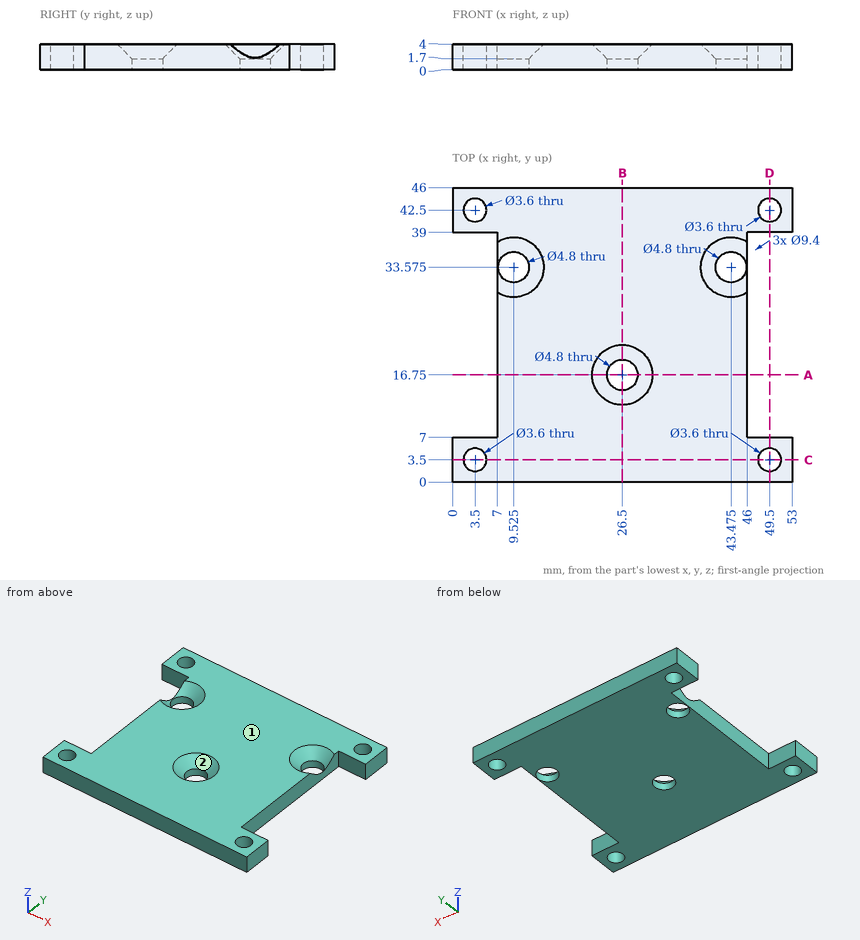
For this review, use the dimensioned drawing (mm, ordinates from the lowest corner) and the shaded views. Coordinates: 2 decimals unless noted, no trailing zeros. Loops run counter-clockwise (first coordinate to the right, second up) from the corner with the lowest first, then second, coordinate; pieces in that order, holes last.
1. For line 1 (Y direction, x = 3.5, z = 0.8); line 2 (X direction, y = 42.5, z = 1.25); line 3 (X direction, y = 4.5, z = 1.8), list the stretches that pass through material, from the lowest coordinate up.
2. Add section D-D, the plane x = 49.5. Give the boundary of the cut face in (y, z).
3. Insertion check: P1, Ø1.2, axis at y = 20.5, z = 2, coming from the +X side; P2, Ø2, axis at y = 27, z = 1.5, coming from the -X side. Each pin has a flat end and moves straight along its axis. Give the tip position at first contact, or say it passes through.
4. Mouldability with a two-part tool opening along Y and no side actions: class the marked faces 1 and 2 as +Y half, -Y half, draft (parallel to the pull), parting line (faces both ways), or undercut.
5. Add section C-C, the plane y = 3.5. Give the boundary of the cut face in (x, z), then the cut area to 3 significant figures.
6. Add section B-B, the plane x = 26.5. Give the boundary of the cut face in (y, z).
7. Add section A-A, the plane y = 16.75. Give the boundary of the cut face in (x, z).
Result:
1. line 1: y = 0 to 1.7, 5.3 to 7, 39 to 40.7, 44.3 to 46
1. line 2: x = 0 to 1.7, 5.3 to 47.7, 51.3 to 53
1. line 3: x = 0 to 2, 5 to 48, 51 to 53
2. outline: (0, 0) - (1.7, 0) - (1.7, 4) - (0, 4) - close; (5.3, 0) - (7, 0) - (7, 4) - (5.3, 4) - close; (39, 0) - (40.7, 0) - (40.7, 4) - (39, 4) - close; (44.3, 0) - (46, 0) - (46, 4) - (44.3, 4) - close
3. P1: stops at x = 46
3. P2: stops at x = 7
4. face 1: draft
4. face 2: undercut
5. outline: (0, 0) - (1.7, 0) - (1.7, 4) - (0, 4) - close; (5.3, 0) - (47.7, 0) - (47.7, 4) - (5.3, 4) - close; (51.3, 0) - (53, 0) - (53, 4) - (51.3, 4) - close
5. area: 183 mm2
6. outline: (0, 0) - (14.35, 0) - (14.35, 1.7) - (12.05, 4) - (0, 4) - close; (19.15, 0) - (46, 0) - (46, 4) - (21.45, 4) - (19.15, 1.7) - close
7. outline: (7, 0) - (24.1, 0) - (24.1, 1.7) - (21.8, 4) - (7, 4) - close; (28.9, 0) - (46, 0) - (46, 4) - (31.2, 4) - (28.9, 1.7) - close
